from build123d import *

# Parameters (mm, degrees)
EXTRUDE_1_DEPTH      = 8
FILLET_1_R           = 5
SKETCH_5_W           = 10
SKETCH_5_H           = 5
CUT_EXTRUDE_1_DEPTH  = 10
SKETCH_6_W           = 55
SKETCH_6_H           = 5
EXTRUDE_2_DEPTH      = 8
SKETCH_7_R           = 5
EXTRUDE_3_DEPTH      = 2
HOLE_WIZARD_1_D      = 4.9
HOLE_WIZARD_1_DEPTH  = 4
HOLE_WIZARD_2_D      = 3
HOLE_WIZARD_3_D      = 4.5
HOLE_WIZARD_3_DEPTH  = 2
SKETCH_16_W          = 45
SKETCH_16_H          = 10
CUT_EXTRUDE_4_DEPTH  = 82.018516402
SKETCH_17_W          = 45
SKETCH_17_H          = 45
EXTRUDE_4_DEPTH      = 16
SKETCH_20_W          = 45
SKETCH_20_H          = 45
CUT_EXTRUDE_5_DEPTH  = 8
SKETCH_21_W          = 10
SKETCH_21_H          = 16
EXTRUDE_6_DEPTH      = 10
SKETCH_23_W          = 55
SKETCH_23_H          = 45
CUT_EXTRUDE_6_DEPTH  = 8
SKETCH_24_W          = 35
SKETCH_24_H          = 8
CUT_EXTRUDE_7_DEPTH  = 3
FILLET_5_R           = 2
SKETCH_25_W          = 45
SKETCH_25_H          = 8
CUT_EXTRUDE_8_DEPTH  = 10
FILLET_6_R           = 15
SKETCH_27_W          = 6
SKETCH_27_H          = 10
CUT_EXTRUDE_10_DEPTH = 5
SKETCH_28_W          = 6
SKETCH_28_H          = 3
CUT_EXTRUDE_11_DEPTH = 76.663729752
SKETCH_29_W          = 10
SKETCH_29_H          = 8
EXTRUDE_7_DEPTH      = 6
FILLET_7_R           = 5


with BuildPart() as part:
    # Sketch 1 → Extrude 1 (new body)
    with BuildSketch(Plane(origin=(0, 0, 0), x_dir=(1, 0, 0), z_dir=(0, 1, 0))):
        Polygon((0, 0), (0, 10), (-70, 10), (-70, -40), (-25, -40), (-25, 0), align=None)
    extrude(amount=EXTRUDE_1_DEPTH)

    # Fillet 1
    fillet_1_edges = [part.edges().sort_by_distance(p)[0] for p in [
        (0, 4, 0),
        (0, 4, -10),
    ]]
    fillet(fillet_1_edges, radius=FILLET_1_R - 0.0001)  # a hair under: the kernel refuses the full size

    # Sketch 5 → Cut-Extrude 1 (cut)
    with BuildSketch(Plane(origin=(0, 8, 0), x_dir=(1, 0, 0), z_dir=(0, 1, 0))):
        with Locations((-20, 2.5)):
            Rectangle(SKETCH_5_W, SKETCH_5_H)
    extrude(amount=-CUT_EXTRUDE_1_DEPTH, mode=Mode.SUBTRACT)

    # Sketch 6 → Extrude 2 (add)
    with BuildSketch(Plane(origin=(0, 8, 0), x_dir=(1, 0, 0), z_dir=(0, 1, 0))):
        with Locations((-42.5, 12.5)):
            Rectangle(SKETCH_6_W, SKETCH_6_H)
    extrude(amount=-EXTRUDE_2_DEPTH)

    # Sketch 7 → Extrude 3 (add)
    with BuildSketch(Plane(origin=(0, 8, 0), x_dir=(1, 0, 0), z_dir=(0, 1, 0))):
        with Locations(Location((-5, 5, 0), (0, 0, 270))):
            Circle(SKETCH_7_R)
    extrude(amount=EXTRUDE_3_DEPTH)

    # Hole Wizard 1
    with Locations(Plane(origin=(0, 10, 0), x_dir=(1, 0, 0), z_dir=(0, 1, 0))):
        with Locations((-5, 5)):
            Hole(HOLE_WIZARD_1_D / 2, depth=HOLE_WIZARD_1_DEPTH)

    # Hole Wizard 2 (through all)
    with Locations(Plane(origin=(0, 0, 0), x_dir=(-1, 0, 0), z_dir=(0, -1, 0))):
        with Locations((5, 5)):
            Hole(HOLE_WIZARD_2_D / 2)

    # Hole Wizard 3
    with Locations(Plane(origin=(0, 0, 0), x_dir=(-1, 0, 0), z_dir=(0, -1, 0))):
        with Locations((5, 5)):
            Hole(HOLE_WIZARD_3_D / 2, depth=HOLE_WIZARD_3_DEPTH)

    # Sketch 16 → Cut-Extrude 4 (cut, through all)
    with BuildSketch(Plane(origin=(0, 8, 0), x_dir=(1, 0, 0), z_dir=(0, 1, 0))):
        with Locations((-47.5, -35)):
            Rectangle(SKETCH_16_W, SKETCH_16_H)
    extrude(amount=-CUT_EXTRUDE_4_DEPTH, mode=Mode.SUBTRACT)

    # Sketch 17 → Extrude 4 (add)
    with BuildSketch(Plane.XZ):
        with Locations((-47.5, 7.5)):
            Rectangle(SKETCH_17_W, SKETCH_17_H)
    extrude(amount=EXTRUDE_4_DEPTH)

    # Sketch 20 → Cut-Extrude 5 (cut)
    with BuildSketch(Plane(origin=(0, 8, 0), x_dir=(1, 0, 0), z_dir=(0, 1, 0))):
        with Locations((-47.5, -7.5)):
            Rectangle(SKETCH_20_W, SKETCH_20_H)
    extrude(amount=-CUT_EXTRUDE_5_DEPTH, mode=Mode.SUBTRACT)


with BuildPart() as cut_extrude_5_piece_1:
    # of the separate pieces the step leaves, piece 1, a body of its own (cut_extrude_5_pieces)
    add(part.part.solids().sort_by_distance((-25, 0, 30))[0])



with BuildPart() as cut_extrude_5_piece_2:
    # of the separate pieces the step leaves, piece 2, a body of its own (cut_extrude_5_pieces)
    add(part.part.solids().sort_by_distance((0, 0, -4.9999))[0])


with BuildPart() as cut_extrude_5_piece_1_1:
    add(cut_extrude_5_piece_1.part)

    add(cut_extrude_5_piece_2.part)  # Extrude 6 merges Cut-Extrude 5 piece 2
    # Sketch 21 → Extrude 6 (add)
    with BuildSketch(Plane(origin=(0, 0, -15), x_dir=(-1, 0, 0), z_dir=(0, 0, -1))):
        with Locations((20, -8)):
            Rectangle(SKETCH_21_W, SKETCH_21_H)
    extrude(amount=-EXTRUDE_6_DEPTH)

    # Sketch 23 → Cut-Extrude 6 (cut)
    with BuildSketch(Plane.XZ.offset(16)):
        with Locations((-42.5, 7.5)):
            Rectangle(SKETCH_23_W, SKETCH_23_H)
    extrude(amount=-CUT_EXTRUDE_6_DEPTH, mode=Mode.SUBTRACT)

    # Sketch 24 → Cut-Extrude 7 (cut)
    with BuildSketch(Plane(origin=(-25, 0, 0), x_dir=(0, 0, -1), z_dir=(1, 0, 0))):
        with Locations((-12.5, -4)):
            Rectangle(SKETCH_24_W, SKETCH_24_H)
    extrude(amount=-CUT_EXTRUDE_7_DEPTH, mode=Mode.SUBTRACT)

    # Fillet 5
    fillet_5_edges = [cut_extrude_5_piece_1_1.edges().sort_by_distance(p)[0] for p in [
        (-15, 0, -15),
        (-15, 4, -10),
    ]]
    fillet(fillet_5_edges, radius=FILLET_5_R)

    # Sketch 25 → Cut-Extrude 8 (cut)
    with BuildSketch(Plane.ZY.offset(70)):
        with Locations((7.5, -4)):
            Rectangle(SKETCH_25_W, SKETCH_25_H)
    extrude(amount=-CUT_EXTRUDE_8_DEPTH, mode=Mode.SUBTRACT)

    # Fillet 6
    fillet_6_edges = [cut_extrude_5_piece_1_1.edges().sort_by_distance(p)[0] for p in [
        (-60, -4, 30),
    ]]
    fillet(fillet_6_edges, radius=FILLET_6_R)

    # Sketch 27 → Cut-Extrude 10 (cut)
    with BuildSketch(Plane(origin=(0, -8, 0), x_dir=(-1, 0, 0), z_dir=(0, -1, 0))):
        with Locations((18, 10)):
            Rectangle(SKETCH_27_W, SKETCH_27_H)
    extrude(amount=-CUT_EXTRUDE_10_DEPTH, mode=Mode.SUBTRACT)

    # Sketch 28 → Cut-Extrude 11 (cut, through all)
    with BuildSketch(Plane(origin=(0, 0, -15), x_dir=(-1, 0, 0), z_dir=(0, 0, -1))):
        with Locations((18, -1.5)):
            Rectangle(SKETCH_28_W, SKETCH_28_H)
    extrude(amount=-CUT_EXTRUDE_11_DEPTH, mode=Mode.SUBTRACT)

    # Sketch 29 → Extrude 7 (add)
    with BuildSketch(Plane.ZY.offset(25)):
        with Locations((-10, 4)):
            Rectangle(SKETCH_29_W, SKETCH_29_H)
    extrude(amount=EXTRUDE_7_DEPTH)

    # Fillet 7
    fillet_7_edges = [cut_extrude_5_piece_1_1.edges().sort_by_distance(p)[0] for p in [
        (-31, 8, -10),
    ]]
    fillet(fillet_7_edges, radius=FILLET_7_R)


solid = cut_extrude_5_piece_1_1.part
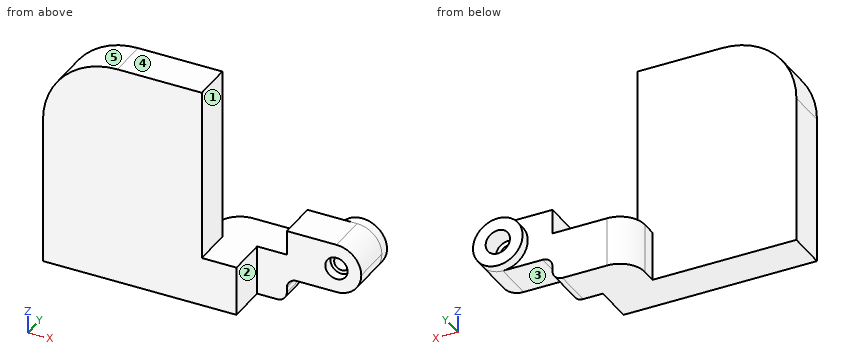
Could you check a few things on this model? Use its own coordinates, in mm. Face numbers are marked on the shaded views. A direction names the side the tool comes from. Coordinates: 2 decimals unless noted, no trailing zeros. Order: outer loops, then holes, each group sorted by start corner. A loop starts at its lowest first (then second) coordinate and runs counter-clockwise, first axis right, second up. Notation, with made-up numbers: (25.5, 62) - (32.5, 62) arc R22 ccw to (32.5, 83) - close; hole circle Ø10 at (58.25, -6.75). An arc over 180 degrees is marked (long way). Answer in a Markdown table with one row per item. Add a question column.
(1) If we section it at C-C, the plane x = -8.5: Please give me the cut outline in (y, z), then the cut area to 3 significant figures.
(2) If we section it at B-B, the plane z = 12: Please give me the cut outline in (x, y).
(3) On a 3-axis mill with a long thin cutter (end or side, diameter ignored), from which of +Z, -Z, +X, -X, +Y, -Y can I reach the whole of each face in a straight line? I mean the marked faces 1, 2, 3, 4 and 5. Say none if no direction works.
(4) Will these pins go through, and if not, where does the flat tip stop? pin 1 (5.5 mm diameter, centred on x = -5, z = -5, fed in from -Y); pin 2 (1.5 mm diameter, centred on y = 2.5, z = -3.5, fed in from -X); pin 3 (6.5 mm diameter, centred on y = -3.5, z = -12, fed in from +X).
(5) If we section it at A-A, the plane y = -1.25: Please give me the cut outline in (x, z).
(6) I need wall thicknesses on L1, parallel to Y at x = -42, z = 25.5; L2, parallel to Z at x = -5, y = 0.5; L3, parallel to Z at x = -25, y = 0. Which ranges of each line are inside material? Lowest first, please.
(7) If we section it at D-D, the plane z = 27: Please give me the cut outline in (x, y).
Results are:
| question | item | result |
|---|---|---|
| 1 | outline | (0, -10) - (8, -10) - (8, -8.57) - (10, -8.57) - (10, -1.43) - (8, -1.43) - (8, 0) - (0, 0) - close |
| 1 | area | 94.3 mm2 |
| 2 | outline | (-60, -8) - (-28, -8) - (-28, 0) - (-60, 0) - close |
| 3 | face 1 | +Z, +X, +Y, -Y |
| 3 | face 2 | +Z, -Z, +X, -Y |
| 3 | face 3 | -Z, +X, +Y, -Y |
| 3 | face 4 | +Z, +X, -X, +Y, -Y |
| 3 | face 5 | +Z, -X, +Y, -Y |
| 4 | pin 1 | stops at y = 0 |
| 4 | pin 2 | stops at x = -15 |
| 4 | pin 3 | stops at x = -21 |
| 5 | outline | (-60, -15) - (-21, -15) - (-21, -5) - (-28, -5) - (-28, 30) - (-45, 30) arc R15 ccw to (-60, 15) - close |
| 6 | L1 | y = -8 to 0 |
| 6 | L2 | z = -10 to -7.25, -2.75 to 0 |
| 6 | L3 | z = -15 to -5 |
| 7 | outline | (-54, -8) - (-28, -8) - (-28, 0) - (-54, 0) - close |
